Design review of the part built by this model. Coordinates are the model's own, in mm. Round coordinates to 2 decimals unless told otherwise and drop trailing zeros. Loops run counter-clockwise (first coordinate to the right, second up) from the corner with the lowest first, then second, coordinate; pieces in that order, holes last. Notation, with made-up numbers: M 12.5,81.5 L 31.5,81.5 A15 ccw 31.5,105.5 Z; hole C 32.25,48.5 d5. An arc over 180 degrees is marked long. One line per item, written item: value. Start each with the question number.
Item 1: We need section D-D (x = 2.5). Write out the cut boundary in (y, z), then the cut area to 3 significant figures.
Item 2: For line 1 along Z through (x, y) = (0, 15.25); line 2 along X through (y, z) = (10.25, -0.75); line 3 along X through (y, z) = (7, -1), list the stretches that pass through material, from the lowest coordinate up.
Item 3: We need section C-C (z = 0.75). Write out the cut boundary in (x, y).
Item 4: Clearance check with a flat-ended pin moving along its axis: pin 1 (1.5 mm diameter, centred on y = 12.5, z = 0.5, fed in from +X). State where the tip first meets the part, or that it passes through.
Item 5: We need section A-A (x = 0). Write out the cut boundary in (y, z).
Item 6: We need section B-B (y = 17.5). Write out the cut boundary in (x, z).
from build123d import *

# Parameters (mm, degrees)
EXTRUDE_1_DEPTH                 = 30
CUT_EXTRUDE_1_REACH             = 32
SKETCH_2_R                      = 2
CUT_EXTRUDE_1_DIRECTION_2_DEPTH = 1


with BuildPart() as part:
    # 草图1 → 凸台-拉伸1 (new body)
    with BuildSketch(Plane(origin=(0, 0, 0), x_dir=(1, 0, 0), z_dir=(0, 1, 0))):
        Polygon((-1.732050808, 3), (1.732050808, 3), (3.464101615, 0), (1.732050808, -3), (-1.732050808, -3), (-3.464101615, 0), align=None)
    extrude(amount=EXTRUDE_1_DEPTH)

    # 草图2 → 切除-拉伸1 (cut, up to next)
    with BuildSketch(Plane(origin=(0, 30, 0), x_dir=(1, 0, 0), z_dir=(0, 1, 0)), mode=Mode.PRIVATE) as cut_extrude_1_sk1:
        Circle(SKETCH_2_R)
    cut_extrude_1_tool1 = extrude(cut_extrude_1_sk1.sketch, amount=-CUT_EXTRUDE_1_REACH, mode=Mode.PRIVATE) & part.part
    add(cut_extrude_1_tool1.solids().sort_by_distance((0, 30, 0))[0], mode=Mode.SUBTRACT)

    # 草图2 → 切除-拉伸1 direction 2 (cut)
    with BuildSketch(Plane(origin=(0, 30, 0), x_dir=(1, 0, 0), z_dir=(0, 1, 0))):
        Circle(SKETCH_2_R)
    extrude(amount=CUT_EXTRUDE_1_DIRECTION_2_DEPTH, mode=Mode.SUBTRACT)


solid = part.part
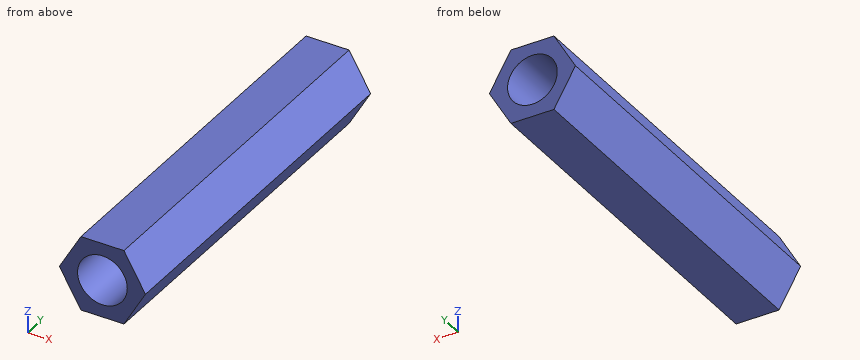
A:
1. outline: M 0,-1.67 L 30,-1.67 L 30,1.67 L 0,1.67 Z
1. area: 100 mm2
2. line 1: -3 to -2, 2 to 3
2. line 2: -3.03 to -1.85, 1.85 to 3.03
2. line 3: -2.89 to -1.73, 1.73 to 2.89
3. outline: M -3.03,0 L -1.85,0 L -1.85,30 L -3.03,30 Z; M 1.85,0 L 3.03,0 L 3.03,30 L 1.85,30 Z
4. pin 1: x = 3.46
5. outline: M 0,-3 L 30,-3 L 30,-2 L 0,-2 Z; M 0,2 L 30,2 L 30,3 L 0,3 Z
6. outline: M -3.46,0 L -1.73,-3 L 1.73,-3 L 3.46,0 L 1.73,3 L -1.73,3 Z; hole C 0,0 d4
